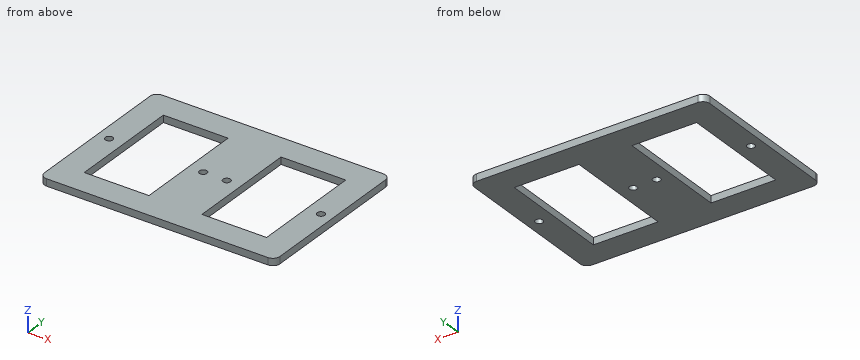
```python
from build123d import *

# Parameters (mm, degrees)
SKETCH1_W            = 100
SKETCH1_H            = 70
SKETCH1_W_2          = 27.5
SKETCH1_H_2          = 48
BOSS_EXTRUDE1_DEPTH  = 3
M3_CLEARANCE_HOLE1_D = 3.2
FILLET1_R            = 3


with BuildPart() as part:
    # Sketch1 → Boss-Extrude1 (new body)
    with BuildSketch(Plane.XY):
        Rectangle(SKETCH1_W, SKETCH1_H)
        with Locations((-25, 0)):
            Rectangle(SKETCH1_W_2, SKETCH1_H_2, mode=Mode.SUBTRACT)
        with Locations((25, 0)):
            Rectangle(SKETCH1_W_2, SKETCH1_H_2, mode=Mode.SUBTRACT)
    extrude(amount=BOSS_EXTRUDE1_DEPTH)

    # M3 Clearance Hole1 (through all)
    with Locations(Plane.XY.offset(3)):
        with Locations((-45, 0), (-5, 0), (45, 0), (5, 0)):
            Hole(M3_CLEARANCE_HOLE1_D / 2)

    # Fillet1
    fillet1_edges = [part.edges().sort_by_distance(p)[0] for p in [
        (-50, 35, 1.5),
        (50, 35, 1.5),
        (50, -35, 1.5),
        (-50, -35, 1.5),
    ]]
    fillet(fillet1_edges, radius=FILLET1_R)


solid = part.part
```
Build history of the part. All positions in model axes, mm. Give positions to 0.01 mm unless a question says otherwise; leave off trailing zeros. Order: outer loops, then holes, each group sorted by start corner. A loop starts at its lowest first (then second) coordinate and runs counter-clockwise, first axis right, second up. Notation, with made-up numbers: M 16,-6.5 L 33,-6.5 A11 ccw 33,13.5 Z; hole C 28.5,72 d7. An arc over 180 degrees is marked long. Return JSON: item names as keys, results as strings.
Q1. Band-saw the part on C-C (y = 0). Give the cut face in (x, z), then the cut area to 3 significant figures.
Answer list:
{"outline": "M -50,0 L -46.6,0 L -46.6,3 L -50,3 Z; M -43.4,0 L -38.75,0 L -38.75,3 L -43.4,3 Z; M -11.25,0 L -6.6,0 L -6.6,3 L -11.25,3 Z; M -3.4,0 L 3.4,0 L 3.4,3 L -3.4,3 Z; M 6.6,0 L 11.25,0 L 11.25,3 L 6.6,3 Z; M 38.75,0 L 43.4,0 L 43.4,3 L 38.75,3 Z; M 46.6,0 L 50,0 L 50,3 L 46.6,3 Z", "area": "96.6 mm^2"}
Q2. Band-saw the part on D-D (z = 1.7). Give the cut face in (x, y).
Answer list:
{"outline": "M -50,-32 A3 ccw -47,-35 L 47,-35 A3 ccw 50,-32 L 50,32 A3 ccw 47,35 L -47,35 A3 ccw -50,32 Z; hole C -45,0 d3.2; hole M -38.75,-24 L -11.25,-24 L -11.25,24 L -38.75,24 Z; hole C -5,0 d3.2; hole C 5,0 d3.2; hole M 11.25,-24 L 38.75,-24 L 38.75,24 L 11.25,24 Z; hole C 45,0 d3.2"}
Q3. Band-saw the part on A-A (y = -8.5). Give the cut face in (x, z), then the cut area to 3 significant figures.
Answer list:
{"outline": "M -50,0 L -38.75,0 L -38.75,3 L -50,3 Z; M -11.25,0 L 11.25,0 L 11.25,3 L -11.25,3 Z; M 38.75,0 L 50,0 L 50,3 L 38.75,3 Z", "area": "135 mm^2"}
Q4. Flat gauge pin, fed straight in: pin 1 (1.9 mm diameter, centred on x = -5, y = 0, fed in from +Z). Where does the tip first touch, or does it go through?
Answer list:
{"pin 1": "passes through"}
Q5. Wall check: probe 1 along X at (y, z) = (4.5, 0.65); probe 2 along Y at (x, z) = (13, 1.5); probe 3 along Y at (x, z) = (-45, 0.95). Give the ranges that are in metal, low to high. Write a range as from..to.
Answer list:
{"probe 1": "x = -50..-38.75, -11.25..11.25, 38.75..50", "probe 2": "y = -35..-24, 24..35", "probe 3": "y = -35..-1.6, 1.6..35"}
Q6. Band-saw the part on B-B (x = -25.5). Give the cut face in (y, z), then the cut area to 3 significant figures.
Answer list:
{"outline": "M -35,0 L -24,0 L -24,3 L -35,3 Z; M 24,0 L 35,0 L 35,3 L 24,3 Z", "area": "66.0 mm^2"}
